Source: CAD feature listing. Evaluate the final solid. Frame: model axes, mm. Round coordinates to 2 decimals unless told otherwise and drop trailing zeros. Loops run counter-clockwise (first coordinate to the right, second up) from the corner with the lowest first, then second, coordinate; pieces in that order, holes last. Notation, with made-up numbers: M 52,64.5 L 57,64.5 A14 ccw 57,76.5 Z; hole C 56.5,45.5 d1. An arc over 180 degrees is marked long. One line per item, written item: value.
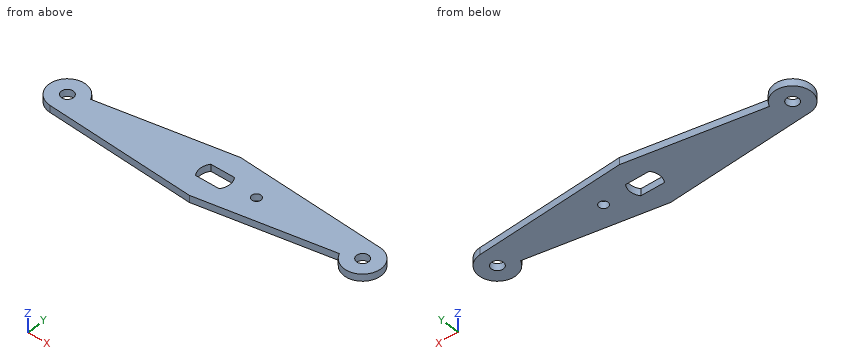
Autodesk Inventor part; units mm, degrees
ref_plane "YZ Plane" through (0, 0, 0) normal (1, 0, 0) x (0, 1, 0)
ref_plane "XZ Plane" through (0, 0, 0) normal (0, 1, 0) x (-1, 0, 0)
ref_plane "XY Plane" through (0, 0, 0) normal (0, 0, 1) x (1, 0, 0)
sketch "Sketch1" plane through (0, 0, 0) normal (0, 0, 1) x (1, 0, 0)
  line L0 (0, 8) -> (0, -8)
  line L1 (0, 8) -> (40.3488, 5.1785)
  arc A0 (35.3957, -1.7588) -> (40.3488, 5.1785) centre (40, 0.1907) ccw
  line L2 (35.3957, -1.7588) -> (0, -8)
  line L3 (0, 0) -> (-17.0336, 0) construction
  dimension "d0" = 16
  dimension "d1" = 10
  dimension "d2" = 14
  dimension "d3" = 40
  dimension "d4" = 10
  dimension "d5" = 7.8093
extrude "Extrusion1" add sketch "Sketch1" along normal blind 1.9
hole "Hole1" at (40, 0.1907, 1.9) direction (0, 0, -1) diameter 3.25 end through all
thread "Thread1"
pattern_circular "Circular Pattern1" count 2 over 360 about axis through (0, 0, -10) along (0, 0, 1)
sketch "Sketch2" plane through (0, 0, 1.9) normal (0, 0, 1) x (1, 0, 0)
  circle A0 centre (0, 0) radius 4
  line L0 (-3.2186, 2.375) -> (3.2186, 2.375)
  line L1 (3.2186, -2.375) -> (-3.2186, -2.375)
  dimension "d20" = 8
  dimension "d21" = 4.75
extrude "Extrusion2" cut sketch "Sketch2" against normal through all contours A0 L1 L0
sketch "Sketch3" plane through (0, 0, 1.9) normal (0, 0, 1) x (1, 0, 0)
  point P0 (0, 0)
  point P1 (10.843, 0.5)
  dimension "d24" = 10.843
  dimension "d25" = 0.5
hole "Hole2" at (10.843, 0.5, 1.9) direction (0, 0, -1) diameter 2.459 end through all
properties part number "406-01" material "Aluminum-6061"
1. Section query D-D (z = 1.4). Count the separate pieces of the cut face and the enclosed holes in it, and give its area (3 significant figures).
Report:
separate pieces: 1
enclosed holes: 4
area: 932 mm2
2. Section query A-A (y = 0.25). Return the cut outline in (x, z).
Report:
outline: M -44.98,0 L -41.56,0 L -41.56,1.9 L -44.98,1.9 Z; M -38.44,0 L -3.99,0 L -3.99,1.9 L -38.44,1.9 Z; M 3.99,0 L 9.64,0 L 9.64,1.9 L 3.99,1.9 Z; M 12.05,0 L 38.38,0 L 38.38,1.9 L 12.05,1.9 Z; M 41.62,0 L 45,0 L 45,1.9 L 41.62,1.9 Z
3. Ray query, line 1 (X direction, y = 0.5, z = 0.8); line 2 (X direction, y = 1, z = 0.6); line 3 (Y direction, x = -34.5, z = 0.35). Return the intervals inside material, ascending. Write a range as [from, to].
Report:
line 1: x = [-44.95, -41.47], [-38.53, -3.97], [3.97, 9.61], [12.07, 38.4], [41.6, 44.99]
line 2: x = [-44.86, -41.11], [-38.89, -3.87], [3.87, 9.72], [11.97, 38.59], [41.41, 44.93]
line 3: y = [-5.59, 1.92]
4. Section query B-B (x = 2). Return the cut outline in (y, z) (3 decimals), and give its area (3 significant figures).
Report:
outline: M -7.647,0 L -2.375,0 L -2.375,1.9 L -7.647,1.9 Z; M 2.375,0 L 7.86,0 L 7.86,1.9 L 2.375,1.9 Z
area: 20.4 mm2
5. Section query C-C (y = 3.75). Return the cut outline in (x, z), and give its area (3 significant figures).
Report:
outline: M -43.08,0 L -36.92,0 L -36.92,1.9 L -43.08,1.9 Z; M -24.1,0 L 43.51,0 L 43.51,1.9 L -24.1,1.9 Z
area: 140 mm2
6. Pin query (flat end, axial travel): pin 1 (0.6 mm diameter, centred on x = -0.5, z = 1.5, fed in from +Y); pin 2 (1 mm diameter, centred on x = 32.5, z = 0.5, fed in from -Y); pin 3 (1 mm diameter, centred on x = -19, z = 0.5, fed in from +Y). Return the tip coordinate at first contact, or that it passes through.
Report:
pin 1: stops at y = 7.96
pin 2: stops at y = -2.36
pin 3: stops at y = 4.74
